Build history of the part. All positions in model axes, mm. Face numbers are marked on the shaded views. A direction names the side the tool comes from. Round coordinates to 2 decimals unless told otherwise and drop trailing zeros. Loops run counter-clockwise (first coordinate to the right, second up) from the corner with the lowest first, then second, coordinate; pieces in that order, holes last.
Autodesk Inventor part; units mm, degrees
ref_plane "YZ Plane" through (0, 0, 0) normal (1, 0, 0) x (0, 1, 0)
ref_plane "XZ Plane" through (0, 0, 0) normal (0, 1, 0) x (-1, 0, 0)
ref_plane "XY Plane" through (0, 0, 0) normal (0, 0, 1) x (1, 0, 0)
sketch "Base" plane through (0, 0, 0) normal (0, 0, 1) x (1, 0, 0)
  line L0 (-45.7522, 47.5316) -> (-101, 9)
  line L1 (44.2478, 47.5316) -> (-45.7522, 47.5316)
  line L2 (-48, 0) -> (-101, 0)
  line L3 (0, 0) -> (-48, 0)
  line L4 (49, 0) -> (0, 0)
  line L5 (74.5, 0) -> (44.2478, 47.5316)
  line L6 (49, 0) -> (74.5, 0)
  line L7 (-101, 0) -> (-101, 9)
  dimension "d29" = 16.3728
  dimension "d30" = 16.3728
  dimension "d48" = 57.525
  dimension "d50" = 145.107
  dimension "d51" = 90
  dimension "d52" = 175.5
  dimension "d53" = 9
  dimension "d57" = 53
  dimension "d58" = 48
  dimension "d59" = 49
extrude "BaseFeature" add sketch "Base" against normal blind 8
fillet "BaseFilletsFeature" radius 2 5 edges at (-101, 9, -4) (-101, 0, -4) (-45.7522, 47.5316, -4) (44.2478, 47.5316, -4) (74.5, 0, -4)
sketch "Sinks" plane through (0, 0, 0) normal (0, 0, 1) x (1, 0, 0)
  line L0 (33.6091, 5) -> (42.4289, 5)
  line L1 (17.2364, 5) -> (7.5711, 5)
  line L2 (17.2364, 5) -> (0.5, 31.2958)
  line L3 (33.6091, 5) -> (49.5, 29.9673)
  line L4 (-32.6091, 5) -> (-41.4289, 5)
  circle A0 centre (0.5, 7.5) radius 7.5
  line L5 (-16.2364, 5) -> (0.5, 31.2958)
  line L6 (-6.5711, 5) -> (-16.2364, 5)
  line L7 (-32.6091, 5) -> (-46.2615, 26.4503)
  circle A1 centre (-85.5, 7.5) radius 7.5
  line L8 (-55.5711, 5) -> (-77.0175, 5)
  line L9 (-46.2615, 26.4503) -> (-77.0175, 5)
  circle A2 centre (-48.5, 7.5) radius 7.5 construction
  line L10 (65.3909, 5) -> (56.5711, 5)
  line L11 (65.3909, 5) -> (49.5, 29.9673)
  circle A3 centre (49.5, 7.5) radius 7.5
  line L12 (37.3455, 42.5316) -> (25.4228, 23.7988)
  line L13 (-12.5, 42.5316) -> (-36.3455, 42.5316)
  line L14 (-24.4228, 23.7988) -> (-12.5, 42.5316)
  line L15 (-24.4228, 23.7988) -> (-36.3455, 42.5316)
  line L16 (13.5, 42.5316) -> (25.4228, 23.7988)
  arc A4 (-41.4289, 5) -> (-55.5711, 5) centre (-48.5, 7.5) ccw
  line L17 (70.8563, 0) -> (-99, 0) construction
  line L18 (-101, 2) -> (-101, 7.9565)
  line L19 (44.8372, 46.6055) -> (72.5436, 3.0739) construction
  line L20 (13.5, 42.5316) -> (37.3455, 42.5316)
  line L21 (-45.1237, 47.5316) -> (43.15, 47.5316) construction
  line L22 (-100.1441, 9.5969) -> (-46.2678, 47.172) construction
  line L23 (0.5, 31.2958) -> (0.5, 7.5) construction
  line L24 (49.5, 29.9673) -> (49.5, 7.5) construction
  point P0 (0, 0)
  point P1 (49.5, 0)
  dimension "d17" = 15
  dimension "d18" = 15.5
  dimension "d19" = 37
  dimension "d20" = 49
  dimension "d21" = 49
  dimension "d22" = 5
  dimension "d23" = 5
  dimension "d24" = 5
  dimension "d25" = 17
  dimension "d26" = 17
  dimension "d27" = 17
  dimension "d28" = 17
  dimension "d29" = 16.3728
  dimension "d30" = 16.3728
  dimension "d32" = 26
  dimension "d33" = 0
  dimension "d35" = 17
extrude "SinksFeature" cut sketch "Sinks" against normal blind 5 contours L3 L11 L10 A3 L0 | L1 A0 L6 L5 L2 | L4 A4 L8 L9 L7 | L12 L16 L20 | L14 L15 L13
fillet "SinkFilletsFeature" radius 2 21 edges at (-46.2615, 26.4503, -2.5) (-77.0175, 5, -2.5) (-32.6091, 5, -2.5) (-55.5711, 5, -2.5) (-41.4289, 5, -2.5) (-36.3455, 42.5316, -2.5) (-12.5, 42.5316, -2.5) (-24.4228, 23.7988, -2.5) (0.5, 31.2958, -2.5) (-16.2364, 5, -2.5) (17.2364, 5, -2.5) (13.5, 42.5316, -2.5) (37.3455, 42.5316, -2.5) (25.4228, 23.7988, -2.5) (49.5, 29.9673, -2.5) (33.6091, 5, -2.5) (65.3909, 5, -2.5) (42.4289, 5, -2.5) (-6.5711, 5, -2.5) (7.5711, 5, -2.5) (56.5711, 5, -2.5)
sketch "Rails" plane through (0, 0, 0) normal (0, 0, 1) x (1, 0, 0)
  line L0 (15.0232, 18.255) -> (5.6268, 33.0184)
  arc A0 (15.0232, 18.255) -> (20.5068, 21.745) centre (17.765, 20) ccw
  line L1 (39.7351, 36.5084) -> (30.3388, 21.745)
  line L2 (35.8223, 18.255) -> (45.2187, 33.0184)
  arc A1 (30.3388, 21.745) -> (35.8223, 18.255) centre (33.0805, 20) ccw
  line L3 (11.1104, 36.5084) -> (20.5068, 21.745)
  arc A2 (45.2187, 33.0184) -> (39.7351, 36.5084) centre (42.4769, 34.7634) ccw
  line L4 (-34.8223, 18.255) -> (-44.2187, 33.0184)
  line L5 (-38.7351, 36.5084) -> (-29.3388, 21.745)
  arc A3 (-34.8223, 18.255) -> (-29.3388, 21.745) centre (-32.0805, 20) ccw
  arc A4 (-38.7351, 36.5084) -> (-44.2187, 33.0184) centre (-41.4769, 34.7634) ccw
  arc A5 (-4.6268, 33.0184) -> (-10.1104, 36.5084) centre (-7.3686, 34.7634) ccw
  line L6 (-14.0232, 18.255) -> (-4.6268, 33.0184)
  line L7 (-10.1104, 36.5084) -> (-19.5068, 21.745)
  arc A6 (-19.5068, 21.745) -> (-14.0232, 18.255) centre (-16.765, 20) ccw
  arc A7 (11.1104, 36.5084) -> (5.6268, 33.0184) centre (8.3686, 34.7634) ccw
  line L8 (-64.9716, 19.8019) -> (-50.6178, 29.8128)
  line L9 (-54.3361, 35.1442) -> (-68.6899, 25.1334)
  arc A8 (-68.6899, 25.1334) -> (-64.9716, 19.8019) centre (-66.8308, 22.4677) ccw
  arc A9 (-50.6178, 29.8128) -> (-54.3361, 35.1442) centre (-52.4769, 32.4785) ccw
  line L10 (-100.1441, 9.5969) -> (-46.2678, 47.172) construction
  line L11 (-71.7978, 8.6404) -> (-47.9727, 25.2568) construction
  line L12 (-45.1413, 24.6903) -> (-34.5656, 8.0739) construction
  line L13 (-26.11, 26.4498) -> (-34.3891, 39.4577) construction
  line L14 (-14.4564, 39.4577) -> (-22.7355, 26.4498) construction
  line L15 (-14.28, 8.0739) -> (-1.1872, 28.6449) construction
  line L16 (2.1872, 28.6449) -> (15.28, 8.0739) construction
  line L17 (23.7355, 26.4498) -> (15.4564, 39.4577) construction
  line L18 (35.3891, 39.4577) -> (27.11, 26.4498) construction
  line L19 (35.5656, 8.0739) -> (47.8128, 27.3164) construction
  line L20 (-32.0805, 20) -> (-16.765, 20) construction
  line L21 (17.765, 20) -> (33.0805, 20) construction
  line L22 (70.8563, 0) -> (-99, 0) construction
  point P0 (0, 0)
  dimension "d29" = 16.3728
  dimension "d30" = 16.3728
  dimension "d36" = 3.25
  dimension "d37" = 17.5
  dimension "d38" = 17
  dimension "d39" = 5.25
  dimension "d40" = 5.25
  dimension "d41" = 5.25
  dimension "d42" = 5.25
  dimension "d43" = 5.25
  dimension "d44" = 5.25
  dimension "d45" = 20
  dimension "d46" = 11
extrude "RailsFeature" cut sketch "Rails" against normal through all
hole "BaseHolesFeature" at (-85.5, 7.5, 0) at (-48.5, 7.5, 0) at (0.5, 7.5, 0) at (49.5, 7.5, 0) direction (0, 0, -1) diameter 6 end through all counterbore diameter 10.5 counterbore depth 4
equation "\"d30\" = d29"
equation "\"d23\" = d22"
equation "\"d24\" = d22"
equation "\"d26\" = d25"
equation "\"d27\" = d25"
equation "\"d28\" = d25"
equation "\"d35\" = d25"
equation "\"d39\" = -d36 + 0.5 * d38"
equation "\"d40\" = d39"
equation "\"d41\" = d39"
equation "\"d42\" = d39"
equation "\"d43\" = d39"
equation "\"d44\" = d39"
properties part number "ForearmUpperShockPlate"
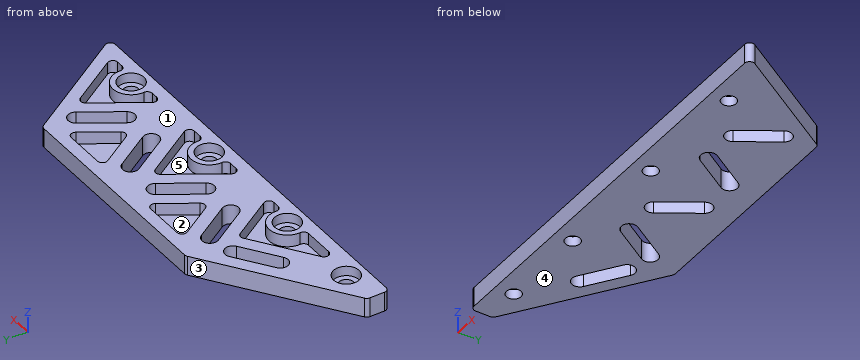
(1) Slice it at A-A on x = 0.5. List the corners of the cut face in (y, z), plus the area to 3 significant figures.
Responses:
outline: (0, -8) - (4.5, -8) - (4.5, -4) - (2.25, -4) - (2.25, 0) - (0, 0) - close; (10.5, -8) - (47.53, -8) - (47.53, 0) - (29.57, 0) - (29.57, -5) - (15, -5) - (15, 0) - (12.75, 0) - (12.75, -4) - (10.5, -4) - close
area: 241 mm2
(2) Pull direction Y, two halves, no side cores. Call the marked faces 1, 2 and 3: +Y half, -Y half, draft (parallel to the pull), parting line (faces both ways), or undercut.
Responses:
face 1: draft
face 2: undercut
face 3: +Y half
(3) Which spindle directions (+Z, -Z, +X, -X, +Y, -Y) get a long thin tool onto all of the face, cutting with end or side? Do the marked faces 4 and 5. Say none if no direction does.
Responses:
face 4: -Z, +X, -X, +Y, -Y
face 5: +Z
(4) Probe line 1 (Y direction, x = 0.5, z = -1.85); line 2 (X direction, y = 17, z = -5.25) (3 decimals); line 3 (Y direction, x = -68.5, z = -0.5). List the from-to ranges inside material, lowest first.
Responses:
line 1: y = 0 to 2.25, 12.75 to 15, 29.57 to 47.53
line 2: x = -89.529 to -33.331, -30.83 to -18.015, -15.515 to 16.515, 19.015 to 31.831, 34.33 to 63.68
line 3: y = 0 to 5, 10.94 to 19.68, 25.27 to 31.67
(5) Slice it at D-D on x = 49.5. List the corners of the cut face in (y, z), plus the area to 3 significant figures.
Responses:
outline: (0, -8) - (4.5, -8) - (4.5, -4) - (2.25, -4) - (2.25, 0) - (0, 0) - close; (10.5, -8) - (39.28, -8) - (39.28, 0) - (28.24, 0) - (28.24, -5) - (15, -5) - (15, 0) - (12.75, 0) - (12.75, -4) - (10.5, -4) - close
area: 182 mm2
(6) Slice it at C-C on x = -85.5. List the corners of the cut face in (y, z).
Responses:
outline: (0, -8) - (4.5, -8) - (4.5, -4) - (2.25, -4) - (2.25, 0) - (0, 0) - close; (10.5, -8) - (19.81, -8) - (19.81, 0) - (12.75, 0) - (12.75, -4) - (10.5, -4) - close
(7) Pin check, flat tips, straight feed: P1, Ø3, axis at x = 60, z = -3.5, coming from the +Y side; P2, Ø5.5, axis at x = -48.5, y = 7.5, coming from the +Z side; P3, Ø1.5, axis at x = -52.5, y = 8.5, coming from the +Z side; P4, Ø1.5, axis at y = 17.5, z = -5, coming from the +X side. Stop position of each tip, or through.
Responses:
P1: stops at y = 25.14
P2: passes through
P3: stops at z = -4
P4: stops at x = 63.84
(8) Slice it at B-B on z = -6.25. Count the separate pieces of the cut face and the enclosed holes in it, plus the area to 3 significant figures.
Responses:
separate pieces: 1
enclosed holes: 9
area: 5,710 mm2
